Geometry check sheet. Reference: the model listing, model coordinates, mm. A direction names the side the tool comes from. Coordinates: 2 decimals unless noted, no trailing zeros. Loops run counter-clockwise (first coordinate to the right, second up) from the corner with the lowest first, then second, coordinate; pieces in that order, holes last.
from build123d import *

# Parameters (mm, degrees)
ESQUISSE1_W             = 10
ESQUISSE1_H             = 10
BOSS_EXTRU_1_DEPTH      = 136
ESQUISSE2_W             = 10
ESQUISSE2_H             = 2
ENL_V_MAT_EXTRU_1_DEPTH = 137.733317081
ESQUISSE3_W             = 10
ESQUISSE3_H             = 10
ENL_V_MAT_EXTRU_2_DEPTH = 2
ESQUISSE4_W             = 10
ESQUISSE4_H             = 10
ENL_V_MAT_EXTRU_3_DEPTH = 2


with BuildPart() as part:
    # Esquisse1 → Boss.-Extru.1 (new body)
    with BuildSketch(Plane.XY):
        with Locations((5, 5)):
            Rectangle(ESQUISSE1_W, ESQUISSE1_H)
    extrude(amount=BOSS_EXTRU_1_DEPTH)

    # Esquisse2 → Enlèv. mat.-Extru.1 (cut, through all)
    with BuildSketch(Plane(origin=(10, 0, 0), x_dir=(0, 0, -1), z_dir=(1, 0, 0))):
        with Locations((-131, 1)):
            Rectangle(ESQUISSE2_W, ESQUISSE2_H)
        with Locations((-78.6, 1)):
            Rectangle(ESQUISSE2_W, ESQUISSE2_H)
        with Locations((-5, 1)):
            Rectangle(ESQUISSE2_W, ESQUISSE2_H)
    extrude(amount=-ENL_V_MAT_EXTRU_1_DEPTH, mode=Mode.SUBTRACT)

    # Esquisse3 → Enlèv. mat.-Extru.2 (cut)
    with BuildSketch(Plane(origin=(10, 0, 0), x_dir=(0, 0, -1), z_dir=(1, 0, 0))):
        with Locations((-40, 5)):
            Rectangle(ESQUISSE3_W, ESQUISSE3_H)
    extrude(amount=-ENL_V_MAT_EXTRU_2_DEPTH, mode=Mode.SUBTRACT)

    # Esquisse4 → Enlèv. mat.-Extru.3 (cut)
    with BuildSketch(Plane(origin=(10, 0, 0), x_dir=(0, 0, -1), z_dir=(1, 0, 0))):
        with Locations((-111, 5)):
            Rectangle(ESQUISSE4_W, ESQUISSE4_H)
    extrude(amount=-ENL_V_MAT_EXTRU_3_DEPTH, mode=Mode.SUBTRACT)


solid = part.part
1) Section check C-C on z = 36.5. Record the cut outline in (x, y).
Data:
outline: (0, 0) - (8, 0) - (8, 10) - (0, 10) - close
2) Section check A-A on x = 1.5. Record the cut outline in (y, z), and give its area (3 significant figures).
Data:
outline: (0, 10) - (2, 10) - (2, 0) - (10, 0) - (10, 136) - (2, 136) - (2, 126) - (0, 126) - (0, 83.6) - (2, 83.6) - (2, 73.6) - (0, 73.6) - close
area: 1,300 mm2
3) Mould release check, pull along Z, two halves, no side actions. Record for faces 6 (the flat face through (5, 2, 79)), 7 (the flat face through (10, 5, 126)), 8 (the flat face through (5, 6, 136)): +Z half, -Z half, draft (parallel to the pull), parting line (faces both ways), or undercut.
Data:
face 6: undercut
face 7: draft
face 8: +Z half
4) Section check B-B on y = 8.5. Record the cut outline in (x, z).
Data:
outline: (0, 0) - (10, 0) - (10, 35) - (8, 35) - (8, 45) - (10, 45) - (10, 106) - (8, 106) - (8, 116) - (10, 116) - (10, 136) - (0, 136) - close
5) Material ranges on probe 1 along Z at (x, y) = (1.5, 0.5); probe 2 along Y at (x, z) = (4.5, 82.5); probe 3 along X at (y, z) = (6.75, 38.5), recorded low to high.
Data:
probe 1: z = 10 to 73.6, 83.6 to 126
probe 2: y = 2 to 10
probe 3: x = 0 to 8
6) Access from +Z, -Z, +X, -X, +Y, -Y to the whole of each face (thin tool, end or side, straight path). Record for faces 1 (the flat face through (5, 2, 131)), 2 (the flat face through (0, 5, 67)), 3 (the flat face through (8, 5, 111)), 4 (the flat face through (5, 2, 5)), 5 (the flat face through (10, 5, 17)).
Data:
face 1: +Z, +X, -X, -Y
face 2: +Z, -Z, -X, +Y, -Y
face 3: +X, +Y, -Y
face 4: -Z, +X, -X, -Y
face 5: +Z, -Z, +X, +Y, -Y
7) Depth check by flat-ended pin: pin 1 (0.6 mm diameter, centred on x = 6.5, y = 1, fed in from -Z); pin 2 (3 mm diameter, centred on x = 7, z = 5, fed in from -Y); pin 3 (5 mm diameter, centred on y = 3.5, z = 40, fed in from +X). Enter the tip coordinate at first touch or a pass-through.
Data:
pin 1: stops at z = 10
pin 2: stops at y = 2
pin 3: stops at x = 8
